Source: CAD feature listing. Evaluate the final solid. Frame: model axes, mm. Face numbers are marked on the shaded views. A direction names the side the tool comes from. Give positions to 0.01 mm unless a question says otherwise; leave off trailing zeros. Write each loop counter-clockwise with the first axis right and the second up, starting at its lowest first coordinate (ties: lowest second). Pieces come first, ordered by that corner, then holes.
```python
from build123d import *

# Parameters (mm, degrees)
F1_DEPTH = 40.64


with BuildPart() as f1:
    # F0 (on Top) → F1 (new body)
    with BuildSketch(Plane.XY):
        with BuildLine():
            Line((0, 45.589266), (0, -20.450734))
            Line((0, -20.450734), (-8.636, -20.450734))
            Line((-8.636, -20.450734), (-8.636, -18.583086))
            Line((-8.636, -18.583086), (-11.811, -20.450734))
            Line((-11.811, -20.450734), (-11.811, -22.318379))
            ThreePointArc((-11.811, -22.318379), (-10.881064, -24.563443), (-8.636, -25.493379))
            Line((-8.636, -25.493379), (0, -25.493379))
            ThreePointArc((0, -25.493379), (2.245064, -24.563443), (3.175, -22.318379))
            Line((3.175, -22.318379), (3.175, -20.450734))
            Line((3.175, -20.450734), (3.175, 45.589266))
            Line((3.175, 45.589266), (8.255, 45.589266))
            Line((8.255, 45.589266), (8.255, 26.165736))
            Line((8.255, 26.165736), (11.43, 26.165736))
            Line((11.43, 26.165736), (11.43, 48.390736))
            ThreePointArc((11.43, 48.390736), (10.500064, 50.6358), (8.255, 51.565736))
            Line((8.255, 51.565736), (3.175, 51.565736))
            Line((3.175, 51.565736), (0, 51.565736))
            Line((0, 51.565736), (-5.461, 51.565736))
            ThreePointArc((-5.461, 51.565736), (-9.951128, 49.705865), (-11.811, 45.215736))
            Line((-11.811, 45.215736), (-11.811, 39.239265))
            Line((-11.811, 39.239265), (-8.636, 39.239265))
            Line((-8.636, 39.239265), (-8.636, 45.589266))
            Line((-8.636, 45.589266), (0, 45.589266))
        make_face()
    extrude(amount=F1_DEPTH)


solid = f1.part
```
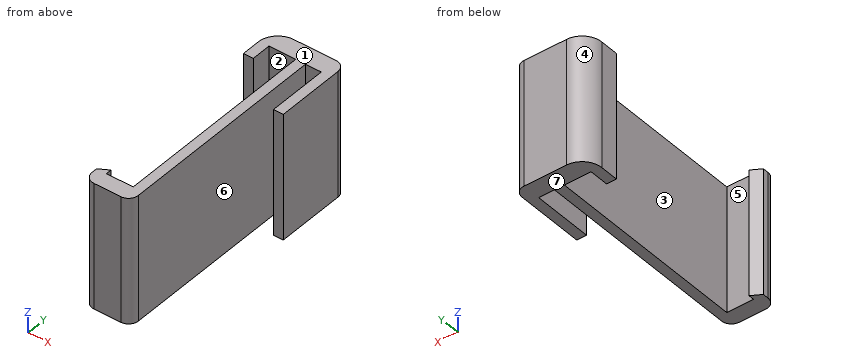
1. Access query for the marked faces 5, 6 and 7. Directions: +Z, -Z, +X, -X, +Y, -Y. A direction counts if a zero-diameter tool reaches every point of the face in a straight line with its end or side. Return the directions, or none.
2. Line query: L1, parallel to X at y = 40.5, z = 11 (3 decimals); L2, parallel to X at y = 34, z = 18 (3 decimals); L3, parallel to Y at x = -3.25, z = 8.5. Output: solid intervals per line, ascending.
3. Cut plane A-A, the plane x = -7.75. Return the cut outline in (y, z), then the cut area to 3 significant figures.
4. Cut plane D-D, the plane y = -9. Return the cut outline in (x, z) (3 decimals), then the cut area to 3 significant figures.
5. Contact query for flat-ended pins moving along their axis: P1, Ø12, axis at y = 4.5, z = 20, coming from the +X side (3 decimals); P2, Ø2, axis at x = 5.5, z = 8, coming from the -Y side; P3, Ø8, axis at y = 5.5, z = 22, coming from the -X side. Output: stop coordinate, or through.
6. Cut plane B-B, the plane z = 7.5. Return the cut outline in (x, y) (3 decimals).
7. Mould query, pull axis Y, two halves, no side actions, for the marked faces 1, 2, 3 and 4. Classes: +Y half, -Y half, draft (parallel to the pull), parting line (faces both ways), or undercut.
8. Cut plane C-C, the plane x = 4.25. Return the cut outline in (y, z), then the cut area to 3 significant figures.
Response values:
1. face 5: +Z, -Z
1. face 6: +Z, -Z, -Y
1. face 7: -Z, +X, -X, +Y, -Y
2. L1: x = -11.811 to -8.636, 0 to 3.175, 8.255 to 11.43
2. L2: x = 0 to 3.175, 8.255 to 11.43
2. L3: y = -25.49 to -20.45, 45.59 to 51.57
3. outline: (-25.49, 0) - (-20.45, 0) - (-20.45, 40.64) - (-25.49, 40.64) - close; (45.59, 0) - (51.14, 0) - (51.14, 40.64) - (45.59, 40.64) - close
3. area: 430 mm2
4. outline: (0, 0) - (3.175, 0) - (3.175, 40.64) - (0, 40.64) - close
4. area: 129 mm2
5. P1: stops at x = 3.175
5. P2: stops at y = 45.59
5. P3: stops at x = 0
6. outline: (-11.811, -22.318) arc R3.175 ccw to (-8.636, -25.493) - (0, -25.493) arc R3.175 ccw to (3.175, -22.318) - (3.175, 45.589) - (8.255, 45.589) - (8.255, 26.166) - (11.43, 26.166) - (11.43, 48.391) arc R3.175 ccw to (8.255, 51.566) - (-5.461, 51.566) arc R6.35 ccw to (-11.811, 45.216) - (-11.811, 39.239) - (-8.636, 39.239) - (-8.636, 45.589) - (0, 45.589) - (0, -20.451) - (-8.636, -20.451) - (-8.636, -18.583) - (-11.811, -20.451) - close
7. face 1: draft
7. face 2: undercut
7. face 3: undercut
7. face 4: +Y half
8. outline: (45.59, 0) - (51.57, 0) - (51.57, 40.64) - (45.59, 40.64) - close
8. area: 243 mm2
